Read the model definition and answer for the solid it produces. Units are mm, in the model's axes. Coordinates: 2 decimals unless noted, no trailing zeros. Loops run counter-clockwise (first coordinate to the right, second up) from the corner with the lowest first, then second, coordinate; pieces in that order, holes last. Notation, with made-up numbers: (-3, 40.25) -> (56, 40.25) arc R8 ccw to (56, 44.25) -> close; hole circle Ø3 at (27.25, -12). An arc over 180 degrees is marked (long way). Answer as a JSON object with one key per item and string values. Group by question number.
1) Section C-C, the plane z = -12 is taken. Give the vertices of the cut face in (x, y).
2) Section B-B, the plane x = 1.5 is taken. Give the vertices of the cut face in (y, z).
3) Consider probe 1 along Y at (x, z) = (0, -24); probe 2 along Z at (x, y) = (4, 5.5); probe 3 along X at (y, z) = (2, 111). Determine where each line is inside the solid, lowest interval first. Write a range as [from, to].
4) Section A-A, the plane y = 0 is taken. Give the vertices of the cut face in (x, z), plus the area to 3 significant figures.
5) Flat-ended cylindrical pins translate along their axes: P1, Ø1, axis at y = -1.5, z = -189, coming from the +X side; P2, Ø2, axis at x = -7, z = 104.5, coming from the -Y side; P3, Ø2, axis at y = -1.5, z = 180.5, coming from the -X side. Find the tip coordinate at first contact, or state that the pin passes through.
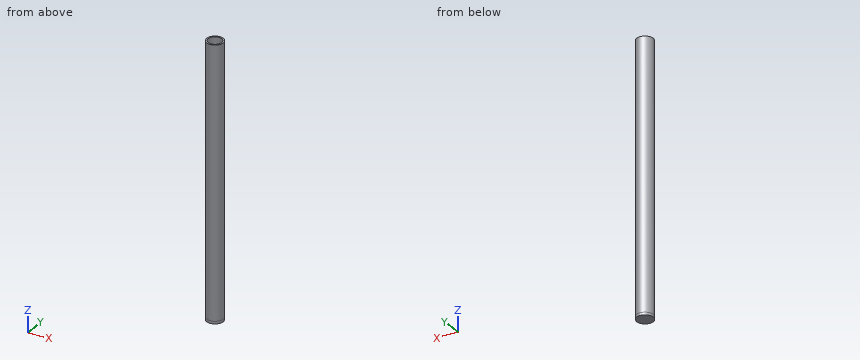
from build123d import *

# Parameters (mm, degrees)
CROQUIS1_R     = 16
EXTRUIR1_DEPTH = 259
VACIADO1_T     = -3
CROQUIS2_R     = 16
EXTRUIR2_DEPTH = 5


with BuildPart() as part:
    # Croquis1 → Extruir1 (new, symmetric)
    with BuildSketch(Plane.XY):
        Circle(CROQUIS1_R)
    extrude(amount=EXTRUIR1_DEPTH, both=True)

    # Vaciado1
    vaciado1_openings = [part.faces().sort_by_distance(p)[0] for p in [
        (0, 0, 259),
        (0, 0, -259),
    ]]
    offset(amount=VACIADO1_T, openings=vaciado1_openings, kind=Kind.INTERSECTION)

    # Croquis2 → Extruir2 (add)
    with BuildSketch(Plane(origin=(0, 0, -259), x_dir=(-1, 0, 0), z_dir=(0, 0, -1))):
        Circle(CROQUIS2_R)
    extrude(amount=EXTRUIR2_DEPTH)


solid = part.part
Determined:
{
 "1": {"outline": "circle Ø32 at (0, 0); hole circle Ø26 at (0, 0)"},
 "2": {"outline": "(-15.93, -264) -> (15.93, -264) -> (15.93, 259) -> (12.91, 259) -> (12.91, -259) -> (-12.91, -259) -> (-12.91, 259) -> (-15.93, 259) -> close"},
 "3": {"probe 1": "[-16, -13], [13, 16]", "probe 2": "[-264, -259]", "probe 3": "[-15.87, -12.85], [12.85, 15.87]"},
 "4": {"outline": "(-16, -264) -> (16, -264) -> (16, 259) -> (13, 259) -> (13, -259) -> (-13, -259) -> (-13, 259) -> (-16, 259) -> close", "area": "3,270 mm²"},
 "5": {"P1": "x = 15.97", "P2": "y = -14.83", "P3": "x = -15.99"}
}
